```python
from build123d import *

# Parameters (mm, degrees)
F0_W     = 43
F0_H     = 43
F1_DEPTH = 5
F2_T     = -1
F4_DEPTH = 4


with BuildPart() as f1:
    # F0 (on Front) → F1 (new body)
    with BuildSketch(Plane.XZ):
        Rectangle(F0_W, F0_H)
    extrude(amount=F1_DEPTH)

    # F2
    f2_openings = [f1.faces().sort_by_distance(p)[0] for p in [
        (0, -2.5, 21.5),
    ]]
    offset(amount=F2_T, openings=f2_openings)

    # F3 (on face) → F4 (cut, through all)
    with BuildSketch(Plane.XZ.offset(5)):
        with BuildLine():
            ThreePointArc((-21.5, 21.5), (-17.9644660941, 20.0355339059), (-16.5, 16.5))
            Line((-16.5, 16.5), (-16.5, -13.5))
            ThreePointArc((-16.5, -13.5), (-15.0355339059, -17.0355339059), (-11.5, -18.5))
            Line((-11.5, -18.5), (11.5, -18.5))
            ThreePointArc((11.5, -18.5), (15.0355339059, -17.0355339059), (16.5, -13.5))
            Line((16.5, -13.5), (16.5, 16.5))
            ThreePointArc((16.5, 16.5), (17.9644660941, 20.0355339059), (21.5, 21.5))
            Line((21.5, 21.5), (-21.5, 21.5))
        make_face()
    extrude(amount=-F4_DEPTH, mode=Mode.SUBTRACT)


solid = f1.part
```
The model under review builds one solid part; all positions refer to its coordinate system, in mm. A direction names the side the tool comes from. Give positions to 0.01 mm unless a question says otherwise; leave off trailing zeros. Write each loop counter-clockwise with the first axis right and the second up, starting at its lowest first coordinate (ties: lowest second). Pieces come first, ordered by that corner, then holes. Notation, with made-up numbers: M 23.25,74.5 L 61.25,74.5 A15 ccw 61.25,92.5 Z; hole C 79,23 d8. An arc over 180 degrees is marked long. Write item = value, one per line. Start each with the question number.
Q1. Mouldability with a two-part tool opening along X and no side actions: class faces 4 (the face through (-21.5, -2, 0)), 5 (the face through (0, 0, 0)), 6 (the face through (0, -1, 1)), 7 (the face through (21.5, -2, 0)) as released by +X, released by -X, zero draft, split by the parting line, or undercut.
Q2. Clearance check with flat-ended pins moving along their axes: pin 1 (1.5 mm diameter, centred on x = -10, y = -4.5, fed in from +Z); pin 2 (20.5 mm diameter, centred on x = -1.5, z = -6.5, fed in from +Y); pin 3 (2.5 mm diameter, centred on x = 1, y = -2.5, fed in from +Z). State where each tip first meets the part, or that it passes through.
Q3. We need section C-C (y = -3.4). State the section outline as (x, z) points.
Q4. We need section B-B (x = 3). State the section outline as (y, z) points, plus the area to 3 significant figures.
Q5. For line 1 (Y direction, x = -17.5, z = -12); line 2 (X direction, y = -2.1, z = 14); line 3 (X direction, y = -4.5, z = 3), list the stretches that pass through material, from the lowest coordinate up.
Q6. Machinability: for faces 1 (the face through (-0.2, -4.5, -18.5)), 2 (the face through (-20.5, -2, 0)), 3 (the face through (0, -5, -19)), which of the approach directions +Z, -Z, +X, -X, +Y, -Y give a long, thin tool a straight path to every point of the face, cutting with its end or side? Answer none if there is none.
Q7. We need section D-D (z = -13). State the section outline as (x, y) points, plus the area to 3 significant figures.
Q8. We need section A-A (z = -19). State the section outline as (x, y) points, plus the area to 3 significant figures.
Result set:
q1.face_4 = released by -X
q1.face_5 = zero draft
q1.face_6 = undercut
q1.face_7 = released by +X
q2.pin_1 = -18.5
q2.pin_2 = 0
q2.pin_3 = -20.5
q3.outline = M -21.5,-21.5 L 21.5,-21.5 L 21.5,21.5 A5 ccw 20.5,21.4 L 20.5,-20.5 L -20.5,-20.5 L -20.5,21.4 A5 ccw -21.5,21.5 Z
q4.outline = M -5,-21.5 L 0,-21.5 L 0,21.5 L -1,21.5 L -1,-20.5 L -4,-20.5 L -4,-18.5 L -5,-18.5 Z
q4.area = 49.0 mm2
q5.line_1 = -5 to -4, -1 to 0
q5.line_2 = -21.5 to -20.5, 20.5 to 21.5
q5.line_3 = -21.5 to -16.5, 16.5 to 21.5
q6.face_1 = +Z, -Y
q6.face_2 = +Z
q6.face_3 = +Z, -Z, +X, -X, -Y
q7.outline = M -21.5,-5 L -16.5,-5 L -16.5,-4 L -20.5,-4 L -20.5,-1 L 20.5,-1 L 20.5,-4 L 16.5,-4 L 16.5,-5 L 21.5,-5 L 21.5,0 L -21.5,0 Z
q7.area = 59.0 mm2
q8.outline = M -21.5,-5 L 21.5,-5 L 21.5,0 L -21.5,0 Z; hole M -20.5,-4 L 20.5,-4 L 20.5,-1 L -20.5,-1 Z
q8.area = 92.0 mm2
